Part model, mm, in its own coordinate system. Give positions to 0.01 mm unless a question says otherwise; leave off trailing zeros. Write each loop counter-clockwise with the first axis right and the second up, starting at its lowest first coordinate (ties: lowest second). Pieces come first, ordered by that corner, then holes.
```python
from build123d import *

# Parameters (mm, degrees)
SKETCH1_W           = 78
SKETCH1_H           = 112
SKETCH1_W_2         = 70.4
SKETCH1_H_2         = 104.4
BOSS_EXTRUDE1_DEPTH = 1.5
SKETCH2_W           = 70.4
SKETCH2_H           = 4
BOSS_EXTRUDE3_DEPTH = 1.5
SKETCH4_R           = 1.05
CUT_EXTRUDE1_DEPTH  = 2.5


with BuildPart() as part:
    # Sketch1 → Boss-Extrude1 (new body)
    with BuildSketch(Plane.XY):
        Rectangle(SKETCH1_W, SKETCH1_H)
        Rectangle(SKETCH1_W_2, SKETCH1_H_2, mode=Mode.SUBTRACT)
    extrude(amount=BOSS_EXTRUDE1_DEPTH)

    # Sketch2 → Boss-Extrude3 (add)
    with BuildSketch(Plane.XY.offset(1.5)):
        Rectangle(SKETCH2_W, SKETCH2_H)
    extrude(amount=-BOSS_EXTRUDE3_DEPTH)

    # Sketch4 → Cut-Extrude1 (cut, through all)
    with BuildSketch(Plane.XY.offset(1.5)):
        with Locations((37, 54)):
            Circle(SKETCH4_R)
        with Locations((23, 0)):
            Circle(SKETCH4_R)
        with Locations((-23, 0)):
            Circle(SKETCH4_R)
        with Locations((-37, -54)):
            Circle(SKETCH4_R)
    extrude(amount=-CUT_EXTRUDE1_DEPTH, mode=Mode.SUBTRACT)


solid = part.part
```
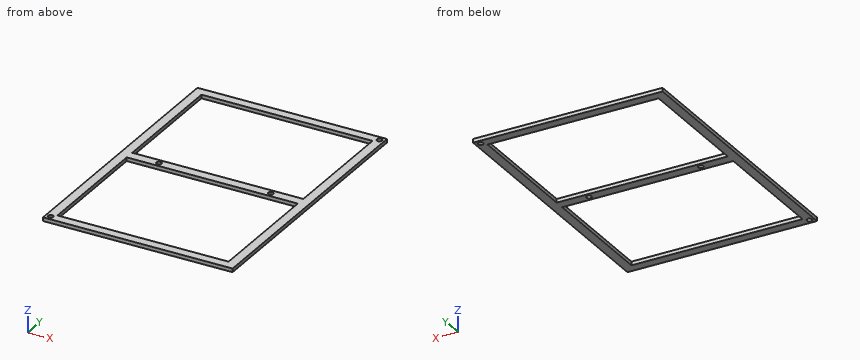
1) Saw through at B-B, the plane x = 17. Write the cut outline in (y, z), then the cut area to 3 significant figures.
Answers follow:
outline: (-56, 0) - (-52.2, 0) - (-52.2, 1.5) - (-56, 1.5) - close; (-2, 0) - (2, 0) - (2, 1.5) - (-2, 1.5) - close; (52.2, 0) - (56, 0) - (56, 1.5) - (52.2, 1.5) - close
area: 17.4 mm2
2) Pin check, flat tip, straight feed: pin 1 Ø1.3 at (x, y) = (37, 54) entering from -Z. Stop position of the tip, or through.
Answers follow:
pin 1: passes through
3) Saw through at A-A, the plane z = 1.2. Write the cut outline in (x, y), then the cut area to 3 significant figures.
Answers follow:
outline: (-39, -56) - (39, -56) - (39, 56) - (-39, 56) - close; hole circle Ø2.1 at (-37, -54); hole (-35.2, -52.2) - (35.2, -52.2) - (35.2, -2) - (-35.2, -2) - close; hole (-35.2, 2) - (35.2, 2) - (35.2, 52.2) - (-35.2, 52.2) - close; hole circle Ø2.1 at (-23, 0); hole circle Ø2.1 at (23, 0); hole circle Ø2.1 at (37, 54)
area: 1,650 mm2
4) Saw through at C-C, the plane y = 32. Write the cut outline in (x, z).
Answers follow:
outline: (-39, 0) - (-35.2, 0) - (-35.2, 1.5) - (-39, 1.5) - close; (35.2, 0) - (39, 0) - (39, 1.5) - (35.2, 1.5) - close
5) Wall check: L1, parallel to Y at x = 23, z = 1.1; L2, parallel to Y at x = 21, z = 0.8; L3, parallel to X at y = -50.5, z = 1.1. Give the ranges that are in metal, low to high.
Answers follow:
L1: y = -56 to -52.2, -2 to -1.05, 1.05 to 2, 52.2 to 56
L2: y = -56 to -52.2, -2 to 2, 52.2 to 56
L3: x = -39 to -35.2, 35.2 to 39
